```python
from build123d import *

# Parameters (mm, degrees)
F0_W      = 50.8
F0_H      = 50.8
F0_W_2    = 44.704000783
F0_H_2    = 44.704000783
F9_DEPTH  = 3.048
F1_W      = 50.8
F1_H      = 50.8
F1_W_2    = 44.704000783
F1_H_2    = 44.704000783
F10_DEPTH = 3.048
F2_W      = 50.8
F2_H      = 50.8
F2_W_2    = 44.704000783
F2_H_2    = 44.704000783
F11_DEPTH = 3.048
F6_W      = 50.8
F6_H      = 50.8
F6_W_2    = 44.704000783
F6_H_2    = 44.704000783
F12_DEPTH = 3.048
F7_W      = 50.8
F7_H      = 50.8
F7_W_2    = 44.704000783
F7_H_2    = 44.704000783
F13_DEPTH = 3.048
F8_W      = 50.8
F8_H      = 50.0440469261
F8_W_2    = 44.7040001482
F8_H_2    = 43.9480470743
F14_DEPTH = 3.048
F15_R     = 3.04799


# Not quite as in the source:
# - a fillet or chamfer is up to 0.001 mm smaller than in the source, because OpenCascade refuses the exact size


with BuildPart() as f9:
    # F0 (on Top) → F9 (new body)
    with BuildSketch(Plane.XY):
        with Locations((25.4, 25.4)):
            Rectangle(F0_W, F0_H)
        with Locations((25.4, 25.4)):
            Rectangle(F0_W_2, F0_H_2, mode=Mode.SUBTRACT)
    extrude(amount=F9_DEPTH)

    # F1 (on Front) → F10 (join)
    with BuildSketch(Plane.XZ):
        with Locations((25.4, 25.4)):
            Rectangle(F1_W, F1_H)
        with Locations((25.4, 25.4)):
            Rectangle(F1_W_2, F1_H_2, mode=Mode.SUBTRACT)
    extrude(amount=-F10_DEPTH)

    # F2 (on Right) → F11 (join)
    with BuildSketch(Plane.YZ):
        with Locations((25.4, 25.4)):
            Rectangle(F2_W, F2_H)
        with Locations((25.4, 25.4)):
            Rectangle(F2_W_2, F2_H_2, mode=Mode.SUBTRACT)
    extrude(amount=F11_DEPTH)

    # F6 (on offset) → F12 (join)
    with BuildSketch(Plane.YZ.offset(50.8)):
        with Locations((25.4, 25.4)):
            Rectangle(F6_W, F6_H)
        with Locations((25.4, 25.4)):
            Rectangle(F6_W_2, F6_H_2, mode=Mode.SUBTRACT)
    extrude(amount=-F12_DEPTH)

    # F7 (on offset) → F13 (join)
    with BuildSketch(Plane.XZ.offset(-50.8)):
        with Locations((25.4, 25.4)):
            Rectangle(F7_W, F7_H)
        with Locations((25.4, 25.4)):
            Rectangle(F7_W_2, F7_H_2, mode=Mode.SUBTRACT)
    extrude(amount=F13_DEPTH)

    # F8 (on offset) → F14 (join)
    with BuildSketch(Plane.XY.offset(50.8)):
        with Locations((25.4, 25.022023463)):
            Rectangle(F8_W, F8_H)
        with Locations((25.4, 25.022023463)):
            Rectangle(F8_W_2, F8_H_2, mode=Mode.SUBTRACT)
    extrude(amount=-F14_DEPTH)

    # F15 (radius 3.048 in the source; OpenCascade refuses exactly that, so slightly less here)
    f15_edges = [f9.edges().sort_by_distance(p)[0] for p in [
        (50.8, 50.8, 25.4),
        (25.4, 50.8, 0),
        (50.8, 25.4, 0),
        (25.4, 0, 0),
        (50.8, 0, 25.4),
        (50.8, 25.4, 50.8),
        (25.4, 50.8, 50.8),
        (25.4, 0, 50.8),
        (0, 25.4, 50.8),
        (0, 50.8, 25.4),
        (0, 25.4, 0),
        (0, 0, 25.4),
    ]]
    fillet(f15_edges, radius=F15_R)


solid = f9.part
```
The listing builds one solid part. Answer for the finished solid, in the listing's coordinates (mm). A direction names the side the tool comes from. Give positions to 0.01 mm unless a question says otherwise; leave off trailing zeros.
1) Consider line 1 along Y through (x, z) = (21, 3); line 2 along Z through (x, y) = (36.5, 49.5). Determine where each line is inside the solid, lowest interval first.
Reported:
line 1: y = 0 to 3.05, 47.75 to 50.8
line 2: z = 0.55 to 3.05, 47.75 to 50.25
2) Given P1, Ø8, axis at y = 8.5, z = 34, coming from the +X side (1 decimal); P2, Ø0.9, axis at x = 1.5, z = 22, coming from the +Y side; P3, Ø1.5, axis at x = 49, y = 35, coming from the +Z side; P4, Ø0.9, axis at x = 49, z = 26, coming from the +Y side, each flat-ended and moving along its own axis, determine where each tip first touches the part or whether it passes through.
Reported:
P1: passes through
P2: stops at y = 50.6
P3: stops at z = 50.76
P4: stops at y = 50.69
3) Determine the mould class of faces 1 (the face through (49.931, 49.883, 25.087)), 2 (the face through (0.869, 25.713, 0.917)), 3 (the face through (49, 3.048, 26)), 4 (the face through (25.713, 49.931, 49.883)) for opening direction Z: pulls with the +Z half, pulls with the -Z half, needs draft (parallel to the pull), parting line crosses it, or undercut.
Reported:
face 1: needs draft
face 2: pulls with the -Z half
face 3: undercut
face 4: pulls with the +Z half
4) For faces 5 (the face through (3.048, 25, 49)), 6 (the face through (25, 2, 3.048)), 7 (the face through (49, 47.752, 25)), determine the directions among +Z, -Z, +X, -X, +Y, -Y from which every point of the face is accessible in a straight line to the end or side of a thin tool.
Reported:
face 5: +Z, -Z
face 6: +Y, -Y
face 7: +X, -X
5) Find section A-A on y = 7.5. Give the number of separate pieces and of enclosed holes in the cut face, then the cut area to 3 significant figures.
Reported:
separate pieces: 4
enclosed holes: 0
area: 29.2 mm2
